Autodesk Inventor part; units mm, degrees
ref_plane "YZ Plane" through (0, 0, 0) normal (1, 0, 0) x (0, 1, 0)
ref_plane "XZ Plane" through (0, 0, 0) normal (0, 1, 0) x (-1, 0, 0)
ref_plane "XY Plane" through (0, 0, 0) normal (0, 0, 1) x (1, 0, 0)
sketch "Sketch1" plane through (0, 0, 0) normal (0, 1, 0) x (-1, 0, 0)
  line L0 (0, 0) -> (6, 0)
  line L1 (6, 0) -> (6, -22)
  line L2 (6, -22) -> (0, -22)
  line L3 (0, -22) -> (0, 0)
  line L4 (9, 3) -> (-3, 3)
  line L5 (-3, 3) -> (-3, -25)
  line L6 (-3, -25) -> (9, -25)
  line L7 (9, -25) -> (9, 3)
  point P0 (3, 0)
  point P1 (3, -25)
  dimension "d0" = 22
  dimension "d1" = 6
  dimension "d2" = 3
  dimension "d3" = 3
  dimension "d4" = 3
  dimension "d5" = 3
extrude "Extrusion1" add sketch "Sketch1" along normal blind 30
sketch "Sketch2" plane through (3, 0, 3) normal (1, 0, 0) x (0, 0, -1)
  circle A0 centre (14, 25) radius 2.75
  line L0 (0, 30) -> (28, 30)
  point P0 (3, 0)
  dimension "d8" = 5.5
  dimension "d11" = 5
extrude "Extrusion2" cut sketch "Sketch2" against normal blind 30
sketch "Sketch3" plane through (3, 0, 3) normal (1, 0, 0) x (0, 0, -1)
  line L0 (6.6175, 3.6795) -> (3.938, 8.3205)
  line L1 (3.938, 8.3205) -> (3.938, 13.6795)
  line L2 (3.938, 13.6795) -> (6.6175, 18.3205)
  line L3 (6.6175, 18.3205) -> (11.2585, 21)
  line L4 (11.2585, 21) -> (16.6175, 21)
  line L5 (16.6175, 21) -> (21.2585, 18.3205)
  line L6 (21.2585, 18.3205) -> (23.938, 13.6795)
  line L7 (23.938, 13.6795) -> (23.938, 8.3205)
  line L8 (23.938, 8.3205) -> (21.2585, 3.6795)
  line L9 (21.2585, 3.6795) -> (16.6175, 1)
  line L10 (16.6175, 1) -> (11.2585, 1)
  line L11 (11.2585, 1) -> (6.6175, 3.6795)
  line L12 (0, 30) -> (28, 30)
  circle A0 centre (14, 10.8347) radius 3.253
  point P0 (3, 0)
  point P1 (13.938, 11)
  dimension "d12" = 10
  dimension "d13" = 19
extrude "Extrusion3" add sketch "Sketch3" along normal blind 10
sketch "Sketch5" plane through (3, 10.8347, -11) normal (1, 0, 0) x (0, 0, -1)
  circle A0 centre (0, 0) radius 1.5
  point P0 (-11, -10.8347)
  dimension "d18" = 3
extrude "Extrusion5" cut sketch "Sketch5" against normal blind 12
properties part number "RollX" material "Thermoplastic Resin"
Here's how the part is built. I have some questions about the finished solid (model axes, mm). A direction names the side the tool comes from. Round coordinates to 2 decimals unless told otherwise and drop trailing zeros. Order: outer loops, then holes, each group sorted by start corner. A loop starts at its lowest first (then second) coordinate and runs counter-clockwise, first axis right, second up. Notation, with made-up numbers: M 22.25,-2.5 L 46.25,-2.5 A16 cw 46.25,16.5 Z; hole C -13,-11.5 d5. An arc over 180 degrees is marked long. Answer as CSV lines item,"result".
Item 1: Which directions (+Z, -Z, +X, -X, +Y, -Y) give clear straight access to the entire face, cutting with the end or side of a thin tool? Please do faces 1 (the flat face through (7.9, 16, -19.6)), 2 (the flat face through (8, 21, -11)), 3 (the flat face through (7.93, 2.36, -15.97)), 4 (the flat face through (7.93, 15.97, -2.26)), 5 (the flat face through (0, 15, -11)).
From the geometry:
face 1,"-Z, +X, +Y"
face 2,"+Z, -Z, +X, +Y"
face 3,"-Z, +X, -Y"
face 4,"+Z, +X, +Y"
face 5,"+Y, -Y"
Item 2: We'd pull the mould along X, two halves only. Please class faces 6 (the flat face through (-6, 15, -11)), 7 (the flat face through (3, 9, -12)), 8 (the flat face through (7.93, 19.679, -15.906)), 9 (the flat face through (-9, 15, -11)): +X half, -X half, draft (parallel to the pull), parting line (faces both ways), or undercut.
From the geometry:
face 6,"undercut"
face 7,"+X half"
face 8,"draft"
face 9,"-X half"
Item 3: Imagine slicing it at A-A on x = -0.5. List the corners of the cut face in (y, z) for me, and give its area (3 significant figures).
From the geometry:
outline,"M 0,-25 L 30,-25 L 30,-22 L 0,-22 Z; M 0,0 L 30,0 L 30,3 L 0,3 Z"
area,"180 mm2"
Item 4: Please list where these lines run through material, in increasing order: L1, parallel to Y at x = -7.8, z = -11; L2, parallel to Z at x = -0.5, y = 5; L3, parallel to Y at x = 0.5, z = -12.25. Write a range as [from, to].
From the geometry:
L1,"[0, 9.33], [12.33, 22.25], [27.75, 30]"
L2,"[-25, -22], [0, 3]"
L3,"[0, 10.01], [11.66, 22.55], [27.45, 30]"
Item 5: Imagine slicing it at C-C on z = -11. Give the number of separate pieces and of enclosed holes in the cut face, and give its area (3 significant figures).
From the geometry:
separate pieces,"6"
enclosed holes,"0"
area,"264 mm2"
Item 6: Imagine slicing it at B-B on y = 25. List the corners of the cut face in (x, z) for me.
From the geometry:
outline,"M -9,-25 L 3,-25 L 3,-13.75 L 0,-13.75 L 0,-22 L -6,-22 L -6,-13.75 L -9,-13.75 Z; M -9,-8.25 L -6,-8.25 L -6,0 L 0,0 L 0,-8.25 L 3,-8.25 L 3,3 L -9,3 Z"
Item 7: For pin 1 (4 mm diameter, centred on y = 10.83, z = -11, fed in from +X); pin 2 (4.5 mm diameter, centred on x = 8, z = -10, fed in from -Y); pin 3 (1.6 mm diameter, centred on x = 7, z = -11, fed in from +Y), each with a flat end and sliding along its axis, tell me the tip position at first contact or that it passes through.
From the geometry:
pin 1,"x = 3"
pin 2,"y = 1"
pin 3,"y = 21"
Item 8: Imagine slicing it at D-D on y = 15.5. List the corners of the cut face in (x, z) for me.
From the geometry:
outline,"M -9,-25 L 3,-25 L 3,-19.89 L 13,-19.89 L 13,-1.99 L 3,-1.99 L 3,3 L -9,3 Z; hole M -6,-22 L 0,-22 L 0,0 L -6,0 Z"
